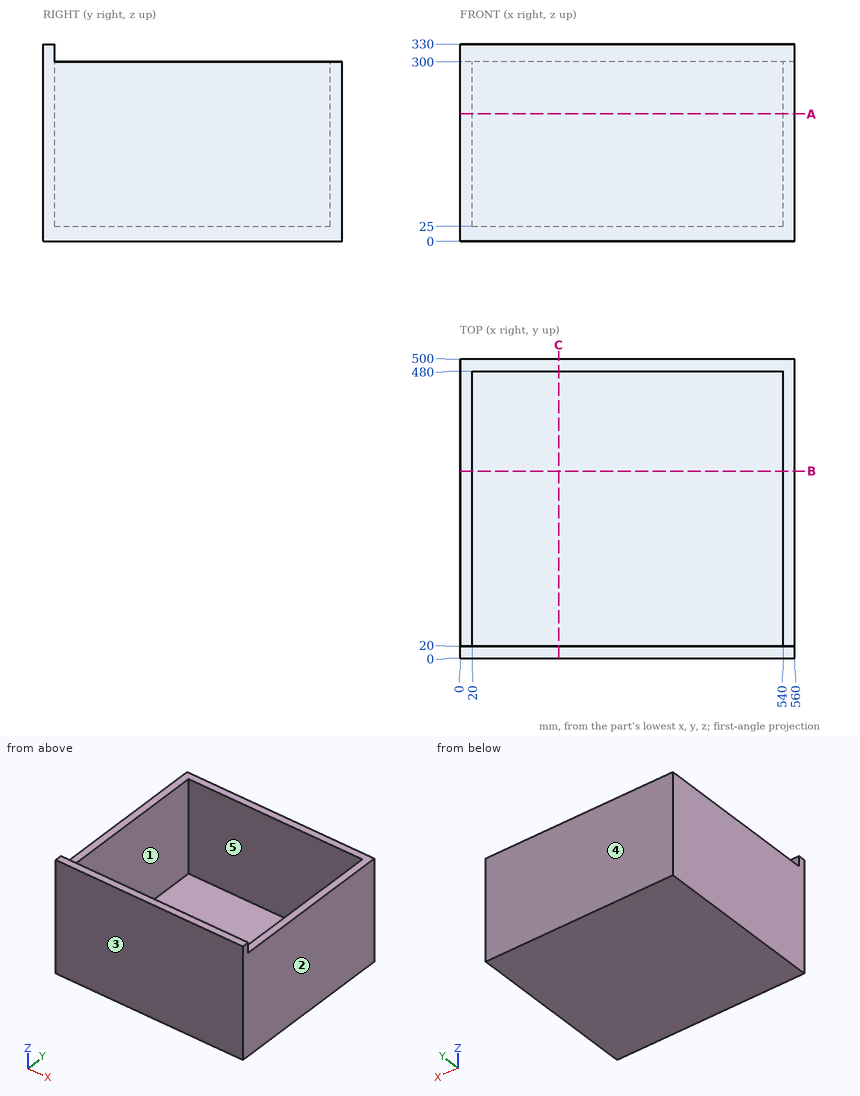
Study the drawing (mm; zero at the part's minimum x, y, z) and answer. A direction names the side the tool comes from. Round coordinates to 2 decimals unless told otherwise and drop trailing zeros. Order: outer loops, then holes, each group sorted by start corner. A loop starts at its lowest first (then second) coordinate and runs counter-clockwise, first axis right, second up. Notation, with made-up numbers: (74, 37.5) - (119, 37.5) arc R16 cw to (119, 57.5) - close; hole circle Ø5 at (-16.75, 47). An arc over 180 degrees is marked (long way). Use one line per item in the form item = value. Start each with the question number.
(1) The part is cut by section A-A (z = 213). Give the vertices of the cut face in (x, y), then the cut area to 3 significant figures.
(2) Determine the mould class of the marked faces 1, 2 and 3 for opening direction Y: +Y half, -Y half, draft (parallel to the pull), parting line (faces both ways), or undercut.
(3) A flat-ended cylindrical pin translates along its axis: pin 1 Ø1.5 at (x, y) = (328, 245) entering from +Z. Find the tip coordinate at first contact, or state that the pin passes through.
(4) The part is cut by section C-C (x = 165). Give the vertices of the cut face in (y, z), then the cut area to 3 significant figures.
(5) Find the intervals of material crossed by line 1 along Y through (x, z) = (36, 40); line 2 along X through (y, z) = (199, 231.5); line 3 along Z through (x, y) = (141.5, 303.5), in increasing order. Write a range as from..to.
(6) The part is cut by section B-B (y = 313). Give the vertices of the cut face in (x, z).
(7) For the marked faces 4 and 5, determine the directions among +Z, -Z, +X, -X, +Y, -Y from which every point of the face is accessible in a straight line to the end or side of a thin tool.
Checked values:
q1.outline = (0, 0) - (560, 0) - (560, 500) - (0, 500) - close; hole (20, 20) - (540, 20) - (540, 480) - (20, 480) - close
q1.area = 40,800 mm^2
q2.face_1 = undercut
q2.face_2 = draft
q2.face_3 = -Y half
q3.pin_1 = 25
q4.outline = (0, 0) - (500, 0) - (500, 300) - (480, 300) - (480, 25) - (20, 25) - (20, 330) - (0, 330) - close
q4.area = 24,100 mm^2
q5.line_1 = 0..20, 480..500
q5.line_2 = 0..20, 540..560
q5.line_3 = 0..25
q6.outline = (0, 0) - (560, 0) - (560, 300) - (540, 300) - (540, 25) - (20, 25) - (20, 300) - (0, 300) - close
q7.face_4 = +Z, -Z, +X, -X, +Y
q7.face_5 = +Z
